Read the model definition and answer for the solid it produces. Units are mm, in the model's axes. Face numbers are marked on the shaded views. A direction names the side the tool comes from. Coordinates: 2 decimals unless noted, no trailing zeros. Write each loop counter-clockwise with the first axis right and the second up, starting at its lowest first coordinate (ties: lowest second). Pieces come first, ordered by that corner, then holes. Notation, with made-up numbers: M -30.75,76.25 L 13.25,76.25 A22 ccw 13.25,83.25 Z; hole C 54,87 d6. An arc over 180 degrees is marked long. Use a Markdown table: item, result. Add a question column.
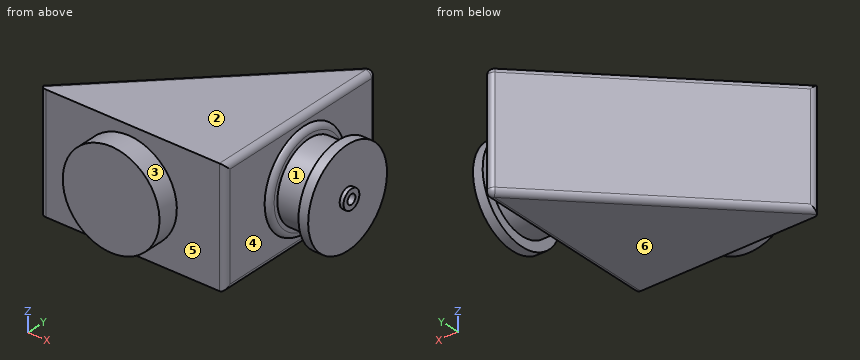
from build123d import *

# Parameters (mm, degrees)
BOSS_EXTRUDE1_DEPTH = 30
FILLET1_R           = 3
SKETCH2_R           = 25
BOSS_EXTRUDE2_DEPTH = 11
SKETCH3_R           = 25
BOSS_EXTRUDE3_DEPTH = 2.5
FILLET2_R           = 3
SKETCH5_R           = 20
BOSS_EXTRUDE4_DEPTH = 15
SKETCH6_R           = 25
BOSS_EXTRUDE5_DEPTH = 5
SKETCH7_R           = 5
BOSS_EXTRUDE6_DEPTH = 2
SKETCH8_R           = 2.5
CUT_EXTRUDE2_DEPTH  = 10


with BuildPart() as part:
    # Sketch1 → Boss-Extrude1 (new, symmetric)
    with BuildSketch(Plane.XY):
        Polygon((0, 0), (100, 0), (100, 100), align=None)
    extrude(amount=BOSS_EXTRUDE1_DEPTH, both=True)

    # Fillet1
    fillet1_edges = [part.edges().sort_by_distance(p)[0] for p in [
        (100, 50, 30),
        (100, 50, -30),
        (50, 50, -30),
        (50, 50, 30),
        (100, 100, 0),
        (100, 0, 0),
        (0, 0, 0),
    ]]
    fillet(fillet1_edges, radius=FILLET1_R)

    # Sketch2 → Boss-Extrude2 (add, symmetric)
    with BuildSketch(Plane.XZ):
        with Locations(Location((50, 0, 0), (0, 0, 90))):
            Circle(SKETCH2_R)
    extrude(amount=BOSS_EXTRUDE2_DEPTH, both=True)

    # Sketch3 → Boss-Extrude3 (add, symmetric)
    with BuildSketch(Plane(origin=(100, 0, 0), x_dir=(0, 0, -1), z_dir=(1, 0, 0))):
        with Locations(Location((0, 50, 0), (0, 0, 180))):
            Circle(SKETCH3_R)
    extrude(amount=BOSS_EXTRUDE3_DEPTH, both=True)

    # Fillet2
    # the kernel refuses this fillet: 3 mm, written as the material it takes off along each edge
    with BuildSketch(Plane(origin=(102.5, 50, 0), x_dir=(0, 0, 1), z_dir=(0, 1, 0))) as fillet2_piece_1:
        with BuildLine():
            CenterArc((22.041960108, -3), FILLET2_R, 9.594068227, 80.405931773)
            Line((22.041960108, 0), (22.041960108, 0.06))
            Line((22.041960108, 0.06), (25, 0.06))
            Line((25, 0.06), (25.06, 0))
            ThreePointArc((25.06, 0), (25.06, -1.25), (25.059160798, -2.49))
            Line((25.059160798, -2.49), (25, -2.5))
        make_face()
    revolve(axis=Axis((102.5, 50, 0), (1, 0, 0)), mode=Mode.SUBTRACT)

    # Sketch5 → Boss-Extrude4 (add)
    with BuildSketch(Plane(origin=(102.5, 0, 0), x_dir=(0, 0, -1), z_dir=(1, 0, 0))):
        with Locations((0, 50)):
            Circle(SKETCH5_R)
    extrude(amount=BOSS_EXTRUDE4_DEPTH)

    # Sketch6 → Boss-Extrude5 (add)
    with BuildSketch(Plane(origin=(117.5, 0, 0), x_dir=(0, 0, -1), z_dir=(1, 0, 0))):
        with Locations((0, 50)):
            Circle(SKETCH6_R)
    extrude(amount=BOSS_EXTRUDE5_DEPTH)

    # Sketch7 → Boss-Extrude6 (add)
    with BuildSketch(Plane(origin=(122.5, 0, 0), x_dir=(0, 0, -1), z_dir=(1, 0, 0))):
        with Locations((0, 50)):
            Circle(SKETCH7_R)
    extrude(amount=BOSS_EXTRUDE6_DEPTH)

    # Sketch8 → Cut-Extrude2 (cut)
    with BuildSketch(Plane(origin=(124.5, 0, 0), x_dir=(0, 0, -1), z_dir=(1, 0, 0))):
        with Locations((0, 50)):
            Circle(SKETCH8_R)
    extrude(amount=-CUT_EXTRUDE2_DEPTH, mode=Mode.SUBTRACT)


solid = part.part
Item 1: For the marked faces 5 and 6, determine the directions among +Z, -Z, +X, -X, +Y, -Y from which every point of the face is accessible in a straight line to the end or side of a thin tool.
Item 2: Each of these flat-tipped pins is pushed along its axis until it touches: pin 1 (6 mm diameter, centred on y = 12.5, z = -3, fed in from +X); pin 2 (4 mm diameter, centred on x = 49.5, z = 16.5, fed in from +Y); pin 3 (6 mm diameter, centred on x = 82, z = 23, fed in from +Y). Where does it stop, or does it pass through?
Item 3: Consider probe 1 along Y at (x, z) = (122, 0); probe 2 along X at (y, z) = (47.5, -2); probe 3 along X at (y, z) = (25, 11). Determine where each line is inside the solid, lowest interval first.
Item 4: Determine the mould class of the marked faces 1, 2, 3 and 4 for opening direction X: pulls with the +X half, pulls with the -X half, needs draft (parallel to the pull), parting line crosses it, or undercut.
Item 5: Find section B-B on y = -3.5. Give the vertices of the cut face in (x, z).
Geometry says:
| question | item | result |
|---|---|---|
| 1 | face 5 | -Y |
| 1 | face 6 | -Z, +X, -X, +Y, -Y |
| 2 | pin 1 | stops at x = 100 |
| 2 | pin 2 | stops at y = 51.5 |
| 2 | pin 3 | stops at y = 85 |
| 3 | probe 1 | y = 25 to 47.5, 52.5 to 75 |
| 3 | probe 2 | x = 47.5 to 124.5 |
| 3 | probe 3 | x = 25 to 100 |
| 4 | face 1 | undercut |
| 4 | face 2 | needs draft |
| 4 | face 3 | parting line crosses it |
| 4 | face 4 | pulls with the +X half |
| 5 | outline | C 50,0 d50 |
